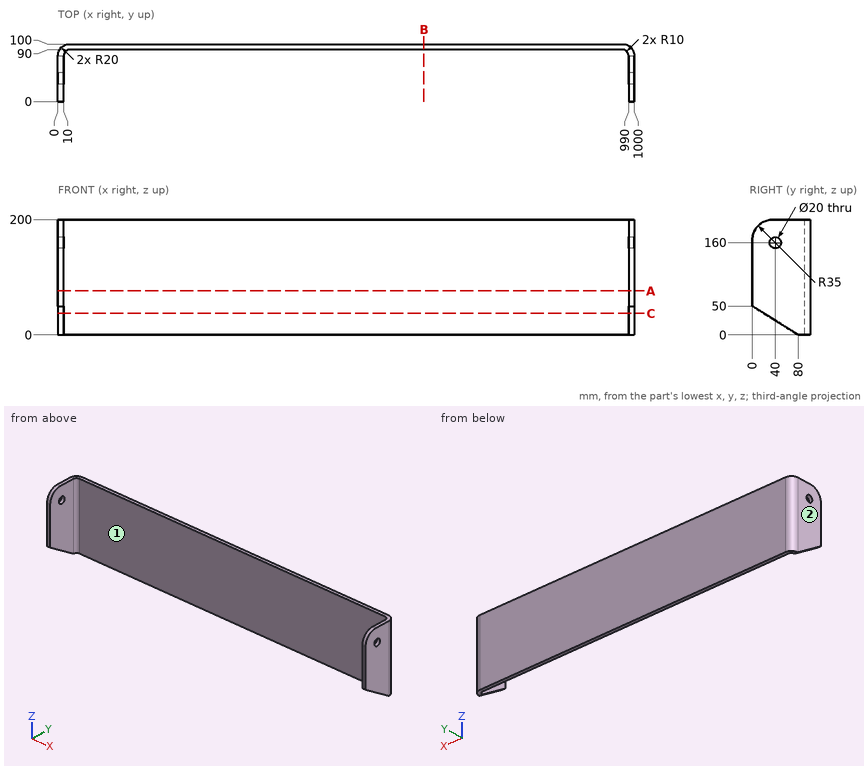
Answer from the drawing. Dimensions are ordinates in mm from the lowest x, y and z of the part. A direction names the side the tool comes from. Coordinates: 2 decimals unless noted, no trailing zeros. Write each loop counter-clockwise with the first axis right and the second up, starting at its lowest first coordinate (ties: lowest second). Pieces come first, ordered by that corner, then holes. Notation, with made-up numbers: (-15.75, -32.75) -> (-7.75, -32.75) arc R22 cw to (-7.75, -10.75) -> close; hole circle Ø5 at (2.25, 42.25). An arc over 180 degrees is marked (long way). One line per question, with ' | ' between items.
1. Straight lines are drawn through the part: line 1 (X direction, y = 46.5, z = 61); line 2 (Y direction, x = 212, z = 96.5); line 3 (Y direction, x = 4.75, z = 160). For each, find the intervals that lie inside material, in ascending order.
Verdict:
line 1: x = 0 to 10, 990 to 1000 | line 2: y = 90 to 100 | line 3: y = 0 to 30, 50 to 92.94
2. Section C-C (z = 37.5) is taken. Determine the outline of the cut face in (x, y).
Verdict:
outline: (0, 20) -> (10, 20) -> (10, 80) arc R10 cw to (20, 90) -> (980, 90) arc R10 cw to (990, 80) -> (990, 20) -> (1000, 20) -> (1000, 80) arc R20 ccw to (980, 100) -> (20, 100) arc R20 ccw to (0, 80) -> close
3. Which of the six approach directions +Z, -Z, +X, -X, +Y, -Y give full straight-line access (tool end or side, diameter ignored) to the marked faces 1 and 2?
Verdict:
face 1: +Z, -Z, -Y | face 2: +Z, -Z, -X, +Y, -Y
4. Section A-A (z = 76.5) is taken. Determine the outline of the cut face in (x, y), and give its area (3 significant figures).
Verdict:
outline: (0, 0) -> (10, 0) -> (10, 80) arc R10 cw to (20, 90) -> (980, 90) arc R10 cw to (990, 80) -> (990, 0) -> (1000, 0) -> (1000, 80) arc R20 ccw to (980, 100) -> (20, 100) arc R20 ccw to (0, 80) -> close | area: 11,700 mm^2
5. Given pin 1 Ø1 at (x, z) = (259, 112) entering from -Y; pin 2 Ø6 at (y, z) = (66.5, 58) entering from -X, each flat-ended and moving along its own axis, determine where each tip first touches the part or whether it passes through.
Verdict:
pin 1: stops at y = 90 | pin 2: stops at x = 0
6. Section B-B (x = 635) is taken. Determine the outline of the cut face in (y, z), and give its area (3 significant figures).
Verdict:
outline: (90, 0) -> (100, 0) -> (100, 200) -> (90, 200) -> close | area: 2,000 mm^2
